The model under review builds one solid part; all positions refer to its coordinate system, in mm. Face numbers are marked on the shaded views. A direction names the side the tool comes from. Coordinates: 2 decimals unless noted, no trailing zeros. Loops run counter-clockwise (first coordinate to the right, second up) from the corner with the lowest first, then second, coordinate; pieces in that order, holes last. Notation, with made-up numbers: M 42.5,28 L 65.5,28 A29 ccw 65.5,57 Z; hole C 32,7.5 d11. An arc over 180 degrees is marked long. Use one line per item in the form item = value.
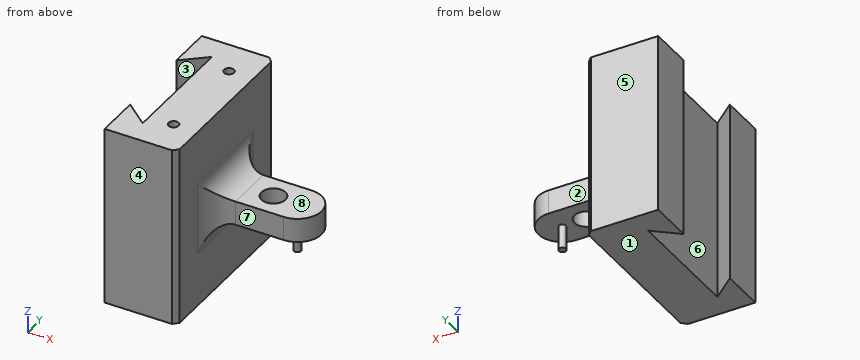
Autodesk Inventor part; units mm, degrees
ref_plane "YZ Plane" through (0, 0, 0) normal (1, 0, 0) x (0, 1, 0)
ref_plane "XZ Plane" through (0, 0, 0) normal (0, 1, 0) x (-1, 0, 0)
ref_plane "XY Plane" through (0, 0, 0) normal (0, 0, 1) x (1, 0, 0)
sketch "Skizze3" plane through (0, 0, 0) normal (0, 0, 1) x (1, 0, 0)
  circle A0 centre (0, 0) radius 5
  circle A1 centre (10, 0) radius 1.5
  line L0 (0, -49) -> (0, 49)
  line L1 (-64, 0) -> (34, 0)
  arc A2 (10, -10) -> (10, 10) centre (10, 0) ccw
  line L2 (10, -10) -> (0, -10)
  line L3 (10, 10) -> (0, 10)
  arc A3 (0, 10) -> (0, -10) centre (0, 0) ccw
  line L4 (0, -10) -> (-20, -10)
  line L5 (0, 10) -> (-20, 10)
  line L6 (-20, -10) -> (-20, -35)
  line L7 (-20, -35) -> (-50, -35)
  line L8 (-50, -35) -> (-50, 35)
  line L9 (-50, 35) -> (-20, 35)
  line L10 (-20, 35) -> (-20, 10)
  line L11 (-50, -16.609) -> (-40, -25)
  line L12 (-40, -25) -> (-40, 25)
  line L13 (-40, 25) -> (-50, 16.609)
  line L14 (-20, -10) -> (-20, 10)
  point P0 (-10, 0)
  dimension "d5" = 10
  dimension "d6" = 3
  dimension "d7" = 10
  dimension "d8" = 20
  dimension "d10" = 10
  dimension "d11" = 50
  dimension "d12" = 30
  dimension "d13" = 20
  dimension "d15" = 25
  dimension "d16" = 25
  dimension "d17" = 10
  dimension "d19" = 50
extrude "Extrusion3" add sketch "Skizze3" along normal mid plane 10 contours L1 A1 A2 L2 L0 A0 | A0 L0 L3 A2 L1 A1 | A0 L1 A3 L0 | L0 A3 L1 A0 | L1 A1 | A1 L1 | A3 L1 L14 L5 | L4 L14 L1 A3
extrude "Extrusion4" add sketch "Skizze3" along normal mid plane 75 contours L14 L1 L12 L13 L8 L9 L10 | L6 L7 L8 L11 L12 L1 L14
chamfer "Fase1" distance 2 angle 45 2 edges at (-20, 35, 0) (-20, -35, 0)
fillet "Rundung1" radius 10 4 edges at (-20, 0, 5) (-20, -10, 0) (-20, 0, -5) (-20, 10, 0)
sketch "Skizze5" plane through (0, 0, 37.5) normal (0, 0, 1) x (1, 0, 0)
  line L0 (-50, -35) -> (-22, -35)
  line L1 (-20, -33) -> (-20, 33)
  line L2 (-22, 35) -> (-50, 35)
  point P0 (0, 0)
  point P1 (-30, 20)
  point P2 (-30, -20)
  dimension "d30" = 15
  dimension "d31" = 10
  dimension "d32" = 15
  dimension "d33" = 10
hole "Bohrung1" at (-30, 20, 37.5) at (-30, -20, 37.5) direction (0, 0, -1) diameter 4.134 depth 15
extrude "Extrusion5" add sketch "Skizze3" against normal blind 15 contours L1 A1 | A1 L1
properties part number "BT401_trajan20_21" material "Kunststoff, undurchsichtig Schwarz"
1. Add section A-A (y = 0). State the section outline as (x, z) points, then the cut area to 3 significant figures.
Response values:
outline = M -40,-37.5 L -20,-37.5 L -20,-15 A10 cw -10,-5 L -5,-5 L -5,5 L -10,5 A10 cw -20,15 L -20,37.5 L -40,37.5 Z; M 5,-5 L 8.5,-5 L 8.5,-15 L 11.5,-15 L 11.5,-5 L 20,-5 L 20,5 L 5,5 Z
area = 1,870 mm^2
2. Add section C-C (z = -16). State the section outline as (x, y) points.
Response values:
outline = M -50,-35 L -22,-35 L -20,-33 L -20,33 L -22,35 L -50,35 L -50,16.61 L -40,25 L -40,-25 L -50,-16.61 Z
3. Insertion check: P1, Ø8, axis at x = 0, y = 0, coming from the -Z side; P2, Ø5, axis at x = 3, z = 0.5, coming from the +Y side; P3, Ø11, axis at x = 2.5, z = -0.5, coming from the -Y side; P4, Ø1.5, axis at y = -22.5, z = -0.5, coming from the +X side. Each pin has a flat end and moves straight along its axis. Give the tip position at first contact, or say it passes through.
Response values:
P1 = through
P2 = 10
P3 = -10
P4 = -20
4. Add section B-B (x = 0). State the section outline as (y, z) points, then the cut area to 3 significant figures.
Response values:
outline = M -10,-5 L -5,-5 L -5,5 L -10,5 Z; M 5,-5 L 10,-5 L 10,5 L 5,5 Z
area = 100 mm^2
5. The part is to be moulded in two halves that separate along Y. For the marked faces 1, 2 and 3, say which applies: pulls with the +Y half, pulls with the -Y half, needs draft (parallel to the pull), parting line crosses it, or undercut.
Response values:
face_1 = needs draft
face_2 = pulls with the +Y half
face_3 = undercut
6. Add section D-D (x = -30). State the section outline as (y, z) points, then the cut area to 3 significant figures.
Response values:
outline = M -35,-37.5 L 35,-37.5 L 35,37.5 L 22.07,37.5 L 22.07,22.5 L 17.93,22.5 L 17.93,37.5 L -17.93,37.5 L -17.93,22.5 L -22.07,22.5 L -22.07,37.5 L -35,37.5 Z
area = 5,130 mm^2
7. Wall thickness on line 1 along Y through (x, z) = (-30, 33); line 2 along X through (y, z) = (-20, 27); line 3 along X through (y, z) = (28.5, 7.5): over which ranges is each line inside the solid? List them lowest first. Write a range as from..to.
Response values:
line_1 = -35..-22.07, -17.93..17.93, 22.07..35
line_2 = -50..-45.96, -40..-32.07, -27.93..-20
line_3 = -50..-20
8. Machinability: for the marked faces 4, 5, 6, 7 and 8, which of the approach directions +Z, -Z, +X, -X, +Y, -Y give a long, thin tool a straight path to every point of the face, cutting with its end or side? Answer none if there is none.
Response values:
face_4 = +Z, -Z, +X, -X, -Y
face_5 = +Z, -Z, +X, -X, +Y
face_6 = +Z, -Z
face_7 = +Z, -Z, +X, -Y
face_8 = +Z, +X, +Y, -Y
